Can you work these out from the model? Positions are in its coordinate system, mm. A direction names the side the tool comes from. Coordinates: 2 decimals unless noted, no trailing zeros. Order: outer loops, then holes, each group sorted by start corner. A loop starts at its lowest first (then second) coordinate and runs counter-clockwise, first axis right, second up. Notation, with made-up numbers: (-24, -32.75) -> (-13, -32.75) arc R15 cw to (-13, -19.75) -> close; hole circle Ø3 at (51, 89). An arc over 180 degrees is marked (long way). Write item = value, one per line.
```python
from build123d import *

# Parameters (mm, degrees)
SKETCH_1_R          = 32.5
SKETCH_1_R_2        = 15
EXTRUDE_1_DEPTH     = 12
SKETCH_2_R          = 1.5
CUT_EXTRUDE_1_DEPTH = 12
EXTRUDE_START       = -12
EXTRUDE_2_DEPTH     = 12
EXTRUDE_3_DEPTH     = 50
SKETCH_5_R          = 3
CUT_EXTRUDE_2_DEPTH = 5
SKETCH_6_R          = 3
CUT_EXTRUDE_3_DEPTH = 3
SKETCH_7_R          = 1.5
CUT_EXTRUDE_9_DEPTH = 105.063682426
FILLET_1_R          = 10


with BuildPart() as part:
    # 草图1 → 凸台-拉伸1 (new body)
    with BuildSketch(Plane(origin=(0, 0, 0), x_dir=(1, 0, 0), z_dir=(0, 1, 0))):
        with Locations(Location((0, 0, 0), (0, 0, 270))):
            Circle(SKETCH_1_R)
        with Locations(Location((0, 0, 0), (0, 0, 270))):
            Circle(SKETCH_1_R_2, mode=Mode.SUBTRACT)
    extrude(amount=EXTRUDE_1_DEPTH)

    # 草图2 → 切除-拉伸1 (cut)
    with BuildSketch(Plane(origin=(0, 12, 0), x_dir=(1, 0, 0), z_dir=(0, 1, 0))):
        with Locations(Location((-15.95, 15.05, 0), (0, 0, 270))):
            Circle(SKETCH_2_R)
        with Locations(Location((15.05, 15.05, 0), (0, 0, 270))):
            Circle(SKETCH_2_R)
        with Locations(Location((15.05, -15.95, 0), (0, 0, 270))):
            Circle(SKETCH_2_R)
        with Locations(Location((-15.95, -15.95, 0), (0, 0, 270))):
            Circle(SKETCH_2_R)
    extrude(amount=-CUT_EXTRUDE_1_DEPTH, mode=Mode.SUBTRACT)

    # 草图3 → 凸台-拉伸2 (add)
    with BuildSketch(Plane(origin=(0, 12, 0), x_dir=(1, 0, 0), z_dir=(0, 1, 0)).offset(EXTRUDE_START)):
        with BuildLine():
            Line((-28.145825623, 50), (-28.145825623, 16.25))
            ThreePointArc((-28.145825623, 16.25), (-16.25, 28.145825623), (0, 32.5))
            Line((0, 32.5), (0, 50))
            Line((0, 50), (-28.145825623, 50))
        make_face()
        with BuildLine():
            ThreePointArc((0, 32.5), (16.25, 28.145825623), (28.145825623, 16.25))
            Line((28.145825623, 16.25), (28.145825623, 50))
            Line((28.145825623, 50), (0, 50))
            Line((0, 50), (0, 32.5))
        make_face()
    extrude(amount=EXTRUDE_2_DEPTH)

    # 草图4 → 凸台-拉伸3 (add)
    with BuildSketch(Plane(origin=(0, 12, 0), x_dir=(1, 0, 0), z_dir=(0, 1, 0))):
        Polygon((28.145825623, 32.5), (28.145825623, 44.5), (-28.145825623, 44.5), (-28.145825623, 32.5), (0, 32.5), align=None)
    extrude(amount=EXTRUDE_3_DEPTH)

    # 草图5 → 切除-拉伸2 (cut)
    with BuildSketch(Plane(origin=(0, 62, 0), x_dir=(1, 0, 0), z_dir=(0, 1, 0))):
        with Locations(Location((0, 38.5, 0), (0, 0, 270))):
            Circle(SKETCH_5_R)
        with Locations(Location((20, 38.5, 0), (0, 0, 270))):
            Circle(SKETCH_5_R)
        with Locations(Location((-20, 38.5, 0), (0, 0, 270))):
            Circle(SKETCH_5_R)
    extrude(amount=-CUT_EXTRUDE_2_DEPTH, mode=Mode.SUBTRACT)

    # 草图6 → 切除-拉伸3 (cut)
    with BuildSketch(Plane.XZ):
        with Locations(Location((15.05, 15.95, 0), (0, 0, 270))):
            Circle(SKETCH_6_R)
        with Locations(Location((-15.95, 15.95, 0), (0, 0, 270))):
            Circle(SKETCH_6_R)
        with Locations(Location((-15.95, -15.05, 0), (0, 0, 270))):
            Circle(SKETCH_6_R)
        with Locations(Location((15.05, -15.05, 0), (0, 0, 270))):
            Circle(SKETCH_6_R)
    extrude(amount=-CUT_EXTRUDE_3_DEPTH, mode=Mode.SUBTRACT)

    # 草图7 → 切除-拉伸9 (cut, through all)
    with BuildSketch(Plane(origin=(0, 0, -44.5), x_dir=(-1, 0, 0), z_dir=(0, 0, -1))):
        with Locations((15.5, 52.5)):
            Circle(SKETCH_7_R)
        with Locations((15.5, 21.5)):
            Circle(SKETCH_7_R)
        with Locations((-15.5, 52.5)):
            Circle(SKETCH_7_R)
        with Locations((-15.5, 21.5)):
            Circle(SKETCH_7_R)
    extrude(amount=-CUT_EXTRUDE_9_DEPTH, mode=Mode.SUBTRACT)

    # 圆角1
    fillet_1_edges = [part.edges().sort_by_distance(p)[0] for p in [
        (0, 0, -50),
    ]]
    fillet(fillet_1_edges, radius=FILLET_1_R)


solid = part.part
```
Item 1: I want a section at B-B, the plane y = 7.5. Please give me the cut outline in (x, z), plus the area to 3 significant figures.
A:
outline = (-28.15, -49.68) -> (28.15, -49.68) -> (28.15, -16.25) arc R32.5 ccw (long way) to (-28.15, -16.25) -> close; hole circle Ø3 at (-15.95, -15.05); hole circle Ø3 at (-15.95, 15.95); hole circle Ø30 at (0, 0); hole circle Ø3 at (15.05, -15.05); hole circle Ø3 at (15.05, 15.95)
area = 3,820 mm2
Item 2: If we mould it in two halves opening along X, with no side actions, what happens to faces 4 (the flat face through (28.146, 24, -37)), 5 (the cylindrical face through (13.586, 7.563, -15.375)), 6 (the cylindrical face through (-0.39, 2.85, -46.99))? For each: pulls with the +X half, pulls with the -X half, needs draft (parallel to the pull), parting line crosses it, or undercut.
A:
face_4 = pulls with the +X half
face_5 = undercut
face_6 = needs draft
Item 3: I want a section at D-D, the plane z = -24. Please give me the cut outline in (x, y), plus the area to 4 significant figures.
A:
outline = (-28.15, 0) -> (28.15, 0) -> (28.15, 12) -> (-28.15, 12) -> close
area = 675.5 mm2
Item 4: If I drill on probe 1 along X at (y, z) = (59.65, -38.5); probe 2 along X at (y, z) = (7, 0); probe 3 along X at (y, z) = (56, -44), over which ranges is the centre line in solid material (lowest first)?
A:
probe_1 = -28.15 to -23, -17 to -3, 3 to 17, 23 to 28.15
probe_2 = -32.5 to -15, 15 to 32.5
probe_3 = -28.15 to 28.15
Item 5: I'm going to push flat-ended pins straight in: P1, Ø1, axis at x = -23, y = 16.5, coming from the -Z side; P2, Ø3, axis at x = -15.5, z = 15, coming from the -Y side; P3, Ø8, axis at x = -15.95, z = -15.05, coming from the +Y side. Where does each tip first touch, or does it pass through?
A:
P1 = -44.5
P2 = 3
P3 = 12
Item 6: I want a section at C-C, the plane x = -25.5. Please give me the cut outline in (y, z).
A:
outline = (0, -40) arc R10 ccw to (10, -50) -> (12, -50) -> (12, -44.5) -> (62, -44.5) -> (62, -32.5) -> (12, -32.5) -> (12, 20.15) -> (0, 20.15) -> close
Item 7: For faces 1 (the cylindrical face through (-19.9, 59.5, -41.5)), 2 (the cylindrical face through (17.58, 1.48, -16.66)), 3 (the cylindrical face through (-17.414, 7.563, -15.375)), which set-ups out of +Z, -Z, +X, -X, +Y, -Y let a thin tool reach every point of the face, with its end or its side?
A:
face_1 = +Y
face_2 = -Y
face_3 = +Y, -Y
Item 8: I want a section at A-A, the plane x = -1.5. Please give me the cut outline in (y, z).
A:
outline = (0, -40) arc R10 ccw to (10, -50) -> (12, -50) -> (12, -44.5) -> (62, -44.5) -> (62, -41.1) -> (57, -41.1) -> (57, -35.9) -> (62, -35.9) -> (62, -32.5) -> (12, -32.5) -> (12, -14.92) -> (0, -14.92) -> close; (0, 14.92) -> (12, 14.92) -> (12, 32.47) -> (0, 32.47) -> close
